from build123d import *

# Parameters (mm, degrees)
SKETCH1_W           = 100
SKETCH1_H           = 48
BOSS_EXTRUDE1_DEPTH = 7
CUT_EXTRUDE1_REACH  = 113.144
SKETCH2_R           = 4.5
SKETCH2_R_2         = 2.2
SKETCH3_W           = 100
SKETCH3_H           = 8
BOSS_EXTRUDE2_DEPTH = 10.2
SKETCH4_R           = 6.6
CUT_EXTRUDE2_DEPTH  = 5.25
SKETCH5_R           = 2.6
CUT_EXTRUDE3_DEPTH  = 7
SKETCH7_R           = 1.5
CUT_EXTRUDE4_DEPTH  = 112.391382072
CUT_EXTRUDE5_REACH  = 114.249
SKETCH8_R           = 1.7
SKETCH9_R           = 3
CUT_EXTRUDE6_DEPTH  = 9
BOSS_EXTRUDE3_DEPTH = 7
CUT_EXTRUDE7_REACH  = 116.246
FILLET1_R           = 10
FILLET2_R           = 10
SKETCH12_R          = 2.6
BOSS_EXTRUDE6_DEPTH = 17.2
FILLET3_R           = 4


with BuildPart() as part:
    # Sketch1 → Boss-Extrude1 (new body)
    with BuildSketch(Plane.XY):
        with Locations((50, 24)):
            Rectangle(SKETCH1_W, SKETCH1_H)
    extrude(amount=BOSS_EXTRUDE1_DEPTH)

    # Sketch2 → Cut-Extrude1 (cut, up to next)
    with BuildSketch(Plane.XY.offset(7), mode=Mode.PRIVATE) as cut_extrude1_sk1:
        with Locations((15, 29)):
            Circle(SKETCH2_R)
    cut_extrude1_tool1 = extrude(cut_extrude1_sk1.sketch, amount=-CUT_EXTRUDE1_REACH, mode=Mode.PRIVATE) & part.part
    # Sketch2 → Cut-Extrude1 (cut, up to next)
    with BuildSketch(Plane.XY.offset(7), mode=Mode.PRIVATE) as cut_extrude1_sk2:
        with Locations((33.75, 29)):
            Circle(SKETCH2_R_2)
    cut_extrude1_tool2 = extrude(cut_extrude1_sk2.sketch, amount=-CUT_EXTRUDE1_REACH, mode=Mode.PRIVATE) & part.part
    # Sketch2 → Cut-Extrude1 (cut, up to next)
    with BuildSketch(Plane.XY.offset(7), mode=Mode.PRIVATE) as cut_extrude1_sk3:
        with Locations((55, 29)):
            Circle(SKETCH2_R_2)
    cut_extrude1_tool3 = extrude(cut_extrude1_sk3.sketch, amount=-CUT_EXTRUDE1_REACH, mode=Mode.PRIVATE) & part.part
    # Sketch2 → Cut-Extrude1 (cut, up to next)
    with BuildSketch(Plane.XY.offset(7), mode=Mode.PRIVATE) as cut_extrude1_sk4:
        with Locations((76.25, 29)):
            Circle(SKETCH2_R_2)
    cut_extrude1_tool4 = extrude(cut_extrude1_sk4.sketch, amount=-CUT_EXTRUDE1_REACH, mode=Mode.PRIVATE) & part.part
    add(cut_extrude1_tool1.solids().sort_by_distance((15, 29, 7))[0], mode=Mode.SUBTRACT)
    add(cut_extrude1_tool2.solids().sort_by_distance((33.75, 29, 7))[0], mode=Mode.SUBTRACT)
    add(cut_extrude1_tool3.solids().sort_by_distance((55, 29, 7))[0], mode=Mode.SUBTRACT)
    add(cut_extrude1_tool4.solids().sort_by_distance((76.25, 29, 7))[0], mode=Mode.SUBTRACT)

    # Sketch3 → Boss-Extrude2 (add)
    with BuildSketch(Plane(origin=(0, 0, 0), x_dir=(-1, 0, 0), z_dir=(0, 0, -1))):
        with Locations((-50, 4)):
            Rectangle(SKETCH3_W, SKETCH3_H)
    extrude(amount=BOSS_EXTRUDE2_DEPTH)

    # Sketch4 → Cut-Extrude2 (cut)
    with BuildSketch(Plane(origin=(0, 0, 0), x_dir=(-1, 0, 0), z_dir=(0, 0, -1))):
        with Locations((-76.25, 29)):
            Circle(SKETCH4_R)
        with Locations((-55, 29)):
            Circle(SKETCH4_R)
        with Locations((-33.75, 29)):
            Circle(SKETCH4_R)
        with Locations((-15, 29)):
            Circle(SKETCH4_R)
    extrude(amount=-CUT_EXTRUDE2_DEPTH, mode=Mode.SUBTRACT)

    # Sketch5 → Cut-Extrude3 (cut)
    with BuildSketch(Plane.XY.offset(7)):
        with Locations((35.000022648, 4.052132501)):
            Circle(SKETCH5_R)
        with Locations((64.999977352, 4)):
            Circle(SKETCH5_R)
    extrude(amount=-CUT_EXTRUDE3_DEPTH, mode=Mode.SUBTRACT)

    # Sketch7 → Cut-Extrude4 (cut, through all)
    with BuildSketch(Plane.XY):
        with Locations((35.000022648, 4.052132501)):
            Circle(SKETCH7_R)
        with Locations((64.999977352, 4)):
            Circle(SKETCH7_R)
    extrude(amount=-CUT_EXTRUDE4_DEPTH, mode=Mode.SUBTRACT)

    # Sketch8 → Cut-Extrude5 (cut, up to next)
    with BuildSketch(Plane.XY.offset(7), mode=Mode.PRIVATE) as cut_extrude5_sk1:
        with Locations((10, 4.052132501)):
            Circle(SKETCH8_R)
    cut_extrude5_tool1 = extrude(cut_extrude5_sk1.sketch, amount=-CUT_EXTRUDE5_REACH, mode=Mode.PRIVATE) & part.part
    # Sketch8 → Cut-Extrude5 (cut, up to next)
    with BuildSketch(Plane.XY.offset(7), mode=Mode.PRIVATE) as cut_extrude5_sk2:
        with Locations((90, 4.052132501)):
            Circle(SKETCH8_R)
    cut_extrude5_tool2 = extrude(cut_extrude5_sk2.sketch, amount=-CUT_EXTRUDE5_REACH, mode=Mode.PRIVATE) & part.part
    add(cut_extrude5_tool1.solids().sort_by_distance((10, 4.052133, 7))[0], mode=Mode.SUBTRACT)
    add(cut_extrude5_tool2.solids().sort_by_distance((90, 4.052133, 7))[0], mode=Mode.SUBTRACT)

    # Sketch9 → Cut-Extrude6 (cut)
    with BuildSketch(Plane.XY.offset(7)):
        with Locations((10, 4.052132501)):
            Circle(SKETCH9_R)
        with Locations((90, 4.052132501)):
            Circle(SKETCH9_R)
    extrude(amount=-CUT_EXTRUDE6_DEPTH, mode=Mode.SUBTRACT)

    # Sketch10 → Boss-Extrude3 (add)
    with BuildSketch(Plane.XY.offset(7)):
        with BuildLine():
            Line((23, 52.5), (58, 52.5))
            ThreePointArc((58, 52.5), (62.5, 48), (58, 43.5))
            Line((58, 43.5), (23, 43.5))
            ThreePointArc((23, 43.5), (18.5, 48), (23, 52.5))
        make_face()
        with BuildLine():
            Line((23, 49.5), (58, 49.5))
            ThreePointArc((58, 49.5), (59.5, 48), (58, 46.5))
            Line((58, 46.5), (23, 46.5))
            ThreePointArc((23, 46.5), (21.5, 48), (23, 49.5))
        make_face(mode=Mode.SUBTRACT)
    extrude(amount=-BOSS_EXTRUDE3_DEPTH)

    # Sketch11 → Cut-Extrude7 (cut, up to next)
    with BuildSketch(Plane.XY.offset(7), mode=Mode.PRIVATE) as cut_extrude7_sk1:
        with BuildLine():
            Line((23, 49.5), (58, 49.5))
            ThreePointArc((58, 49.5), (59.5, 48), (58, 46.5))
            Line((58, 46.5), (23, 46.5))
            ThreePointArc((23, 46.5), (21.5, 48), (23, 49.5))
        make_face()
    cut_extrude7_tool1 = extrude(cut_extrude7_sk1.sketch, amount=-CUT_EXTRUDE7_REACH, mode=Mode.PRIVATE) & part.part
    add(cut_extrude7_tool1.solids().sort_by_distance((40.5, 48, 7))[0], mode=Mode.SUBTRACT)

    # Fillet1
    fillet1_edges = [part.edges().sort_by_distance(p)[0] for p in [
        (0, 48, 3.5),
        (100, 48, 3.5),
    ]]
    fillet(fillet1_edges, radius=FILLET1_R)

    # Fillet2
    fillet2_edges = [part.edges().sort_by_distance(p)[0] for p in [
        (18.5, 48, 3.5),
        (62.5, 48, 3.5),
    ]]
    fillet(fillet2_edges, radius=FILLET2_R)

    # Sketch12 → Boss-Extrude6 (add)
    with BuildSketch(Plane.XY.offset(7)):
        with Locations((35.000022648, 4.052132501)):
            Circle(SKETCH12_R)
        with Locations((64.999977352, 4)):
            Circle(SKETCH12_R)
    extrude(amount=-BOSS_EXTRUDE6_DEPTH)

    # Fillet3
    fillet3_edges = [part.edges().sort_by_distance(p)[0] for p in [
        (50, 8, 0),
    ]]
    fillet(fillet3_edges, radius=FILLET3_R)


solid = part.part
Can you work these out from the model? Positions are in its coordinate system, mm. A direction names the side the tool comes from. Coordinates: 2 decimals unless noted, no trailing zeros. Order: outer loops, then holes, each group sorted by start corner. A loop starts at its lowest first (then second) coordinate and runs counter-clockwise, first axis right, second up. Notation, with made-up numbers: (43, 79.5) - (71, 79.5) arc R16 ccw to (71, 102.5) - close; hole circle Ø7 at (7.5, 16.25). An arc over 180 degrees is marked (long way). Answer as a JSON object with one key per item and string values. Group by question number.
Q1. Imagine slicing it at C-C (x = 64). Please give me the cut outline in (y, z).
Q2. Imagine slicing it at A-A (z = 3.75). Please give me the cut outline in (x, y).
Q3. I need wall thicknesses on line 1 (Y direction, x = 33.75, z = 6.5); line 2 (Y direction, x = 33.75, z = 2.6); line 3 (Y direction, x = 44, z = 1). Which ranges of each line are inside material? Lowest first, please. Write a range as from..to.
Q4. Imagine slicing it at B-B (x = 29). Please give me the cut outline in (y, z).
Q5. On a 3-axis mill with a long thin cutter (end or side, diameter ignored), from which of +Z, -Z, +X, -X, +Y, -Y can I reach the whole of each face in a straight line? I mean faces 1 (the face through (51, 37, 0)), 2 (the face through (12, 4, -2)), 3 (the face through (100, 15, 2)), 4 (the face through (35, 31, 5.25)). Say none if no direction works.
Q6. We'd pull the mould along X, two halves only. Please class faces 5 (the face through (40, 49.5, 4)), 6 (the face through (59.749, 52.146, 3.549)), 7 (the face through (49.3, 9.203, -1.141)): +X half, -X half, draft (parallel to the pull), parting line (faces both ways), or undercut.
Q7. Imagine slicing it at D-D (y = 13). Please give me the cut outline in (x, z), and give its area (3 significant figures).
Q8. Will these pins go through, and if not, where does the flat tip stop? P1, Ø1.8, axis at x = 11.5, y = 2.5, coming from the +Z side; P2, Ø5, axis at x = 26.5, y = 45.5, coming from the -Z side; P3, Ø6.5, axis at x = 13, y = 30, coming from the -Z side; P4, Ø2, axis at x = 11.5, z = 3.5, coming from the +Y side.
Determined:
{
 "1": {"outline": "(0, -10.2) - (8, -10.2) - (8, -4) arc R4 cw to (12, 0) - (49.07, 0) - (49.07, 7) - (0, 7) - close"},
 "2": {"outline": "(0, 0) - (100, 0) - (100, 38) arc R10 ccw to (90, 48) - (68.5, 48) arc R10 cw to (61.26, 51.1) arc R4.5 ccw to (58, 52.5) - (23, 52.5) arc R4.5 ccw to (19.74, 51.1) arc R10 cw to (12.5, 48) - (10, 48) arc R10 ccw to (0, 38) - close; hole circle Ø6 at (10, 4.05); hole circle Ø13.2 at (15, 29); hole (23, 46.5) - (58, 46.5) arc R1.5 ccw to (58, 49.5) - (23, 49.5) arc R1.5 ccw to start; hole circle Ø13.2 at (33.75, 29); hole circle Ø13.2 at (55, 29); hole circle Ø13.2 at (76.25, 29); hole circle Ø6 at (90, 4.05)"},
 "3": {"line 1": "y = 0..26.8, 31.2..46.5, 49.5..52.5", "line 2": "y = 0..22.4, 35.6..46.5, 49.5..52.5", "line 3": "y = 0..46.5, 49.5..52.5"},
 "4": {"outline": "(0, -10.2) - (8, -10.2) - (8, -4) arc R4 cw to (12, 0) - (24.42, 0) - (24.42, 5.25) - (33.58, 5.25) - (33.58, 0) - (46.5, 0) - (46.5, 7) - (0, 7) - close; (49.5, 0) - (52.5, 0) - (52.5, 7) - (49.5, 7) - close"},
 "5": {"face 1": "-Z, +X, -X, +Y", "face 2": "+Z", "face 3": "+Z, -Z, +X, +Y, -Y", "face 4": "-Z"},
 "6": {"face 5": "undercut", "face 6": "+X half", "face 7": "draft"},
 "7": {"outline": "(0, 0) - (100, 0) - (100, 7) - (0, 7) - close", "area": "700 mm2"},
 "8": {"P1": "stops at z = 7", "P2": "stops at z = 0", "P3": "stops at z = 5.25", "P4": "stops at y = 48"}
}
